Read the model definition and answer for the solid it produces. Units are mm, in the model's axes. Face numbers are marked on the shaded views. A direction names the side the tool comes from. Give positions to 0.01 mm unless a question says otherwise; leave off trailing zeros. Loops run counter-clockwise (first coordinate to the right, second up) from the corner with the lowest first, then second, coordinate; pieces in that order, holes last.
(1) Find section B-B, the plane y = -8.5. Write down the section's boundary in (x, z), then the cut area to 3 significant figures.
(2) Which of the six approach directions +Z, -Z, +X, -X, +Y, -Y give full straight-line access (tool end or side, diameter ignored) to the marked faces 4, 5, 6, 7 and 8?
(3) Straight lines are drawn through the part: probe 1 along Y at (x, z) = (4.75, 12.5); probe 2 along Y at (x, z) = (0.5, 6.25); probe 3 along Z at (x, y) = (2.75, -7.75). For each, find the intervals that lie inside material, in ascending order.
(4) Find section C-C, the plane x = 4.5. Write down the section's boundary in (y, z).
(5) Find section D-D, the plane y = 0.5. Write down the section's boundary in (x, z).
(6) Find section A-A, the plane z = 11. Write down the section's boundary in (x, y), then the cut area to 3 significant figures.
(7) Each of these flat-tipped pins is pushed along its axis until it touches: P1, Ø1.8, axis at x = -4.5, z = 4.5, coming from the -Y side; P2, Ø1.5, axis at x = 0.5, y = -3, coming from the -Z side; P3, Ø5, axis at y = 6.5, z = 9.5, coming from the -X side. Where does it stop, or does it pass through?
(8) Determine the mould class of the marked faces 1, 2 and 3 for opening direction Y: pulls with the +Y half, pulls with the -Y half, needs draft (parallel to the pull), parting line crosses it, or undercut.
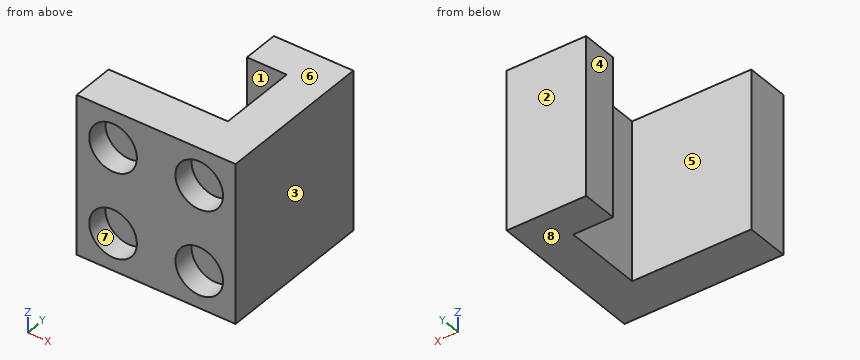
```python
from build123d import *

# Parameters (mm, degrees)
F0_W     = 20
F0_H     = 20
F1_DEPTH = 20
F2_W     = 10
F2_H     = 4.5614074916
F3_DEPTH = 20
F4_R     = 3
F5_DEPTH = 2.75


with BuildPart() as f1:
    # F0 (on Top) → F1 (new body)
    with BuildSketch(Plane.XY):
        Rectangle(F0_W, F0_H)
    extrude(amount=F1_DEPTH)

    # F2 (on face) → F3 (cut)
    with BuildSketch(Plane.XY.offset(20)):
        Polygon((-10, -4.5614074916), (5, -4.5614074916), (5, 5.4385925084), (0, 5.4385925084), (-10, 5.4385925084), align=None)
        with Locations((-5, 7.7192962542)):
            Rectangle(F2_W, F2_H)
    extrude(amount=-F3_DEPTH, mode=Mode.SUBTRACT)

    # F4 (on face) → F5 (cut)
    with BuildSketch(Plane.XZ.offset(10)):
        with Locations((-5.4237376899, 4.6365144663)):
            Circle(F4_R)
        with Locations((-5.4237376899, 15.3634855337)):
            Circle(F4_R)
        with Locations((5.4237376899, 15.3634855337)):
            Circle(F4_R)
        with Locations((5.4237376899, 4.6365144663)):
            Circle(F4_R)
    extrude(amount=-F5_DEPTH, mode=Mode.SUBTRACT)


solid = f1.part
```
Entries:
1. outline: (-10, 0) - (10, 0) - (10, 20) - (-10, 20) - close; hole circle Ø6 at (-5.42, 4.64); hole circle Ø6 at (-5.42, 15.36); hole circle Ø6 at (5.42, 4.64); hole circle Ø6 at (5.42, 15.36)
1. area: 287 mm2
2. face 4: +Z, -Z, -X, +Y
2. face 5: +Z, -Z, -X
2. face 6: +Z, +X, -X, +Y, -Y
2. face 7: -Y
2. face 8: -Z, +X, -X, +Y, -Y
3. probe 1: y = -7.25 to -4.56, 5.44 to 10
3. probe 2: y = -10 to -4.56, 5.44 to 10
3. probe 3: z = 0 to 3.28, 6 to 14, 16.72 to 20
4. outline: (-10, 0) - (-4.56, 0) - (-4.56, 20) - (-10, 20) - (-10, 18.22) - (-7.25, 18.22) - (-7.25, 12.51) - (-10, 12.51) - (-10, 7.49) - (-7.25, 7.49) - (-7.25, 1.78) - (-10, 1.78) - close; (5.44, 0) - (10, 0) - (10, 20) - (5.44, 20) - close
5. outline: (5, 0) - (10, 0) - (10, 20) - (5, 20) - close
6. outline: (-10, -10) - (10, -10) - (10, 10) - (0, 10) - (0, 5.44) - (5, 5.44) - (5, -4.56) - (-10, -4.56) - close
6. area: 204 mm2
7. P1: stops at y = -7.25
7. P2: passes through
7. P3: stops at x = 0
8. face 1: undercut
8. face 2: pulls with the +Y half
8. face 3: needs draft
